```python
from build123d import *

# Parameters (mm, degrees)
F0_R     = 100
F0_R_2   = 16
F1_DEPTH = 60
F2_R     = 5
F2_R_2   = 16
F3_DEPTH = 10


with BuildPart() as f1:
    # F0 (on Right) → F1 (new body)
    with BuildSketch(Plane.YZ):
        Circle(F0_R)
        Circle(F0_R_2, mode=Mode.SUBTRACT)
    extrude(amount=F1_DEPTH)

    # F2 (on face) → F3 (join)
    with BuildSketch(Plane.YZ.offset(60)):
        with BuildLine():
            Line((-83.269003, -55.37394), (-94.310643, -89.356614))
            ThreePointArc((-94.310643, -89.356614), (-90.759655, -111.776671), (-70.53423, -122.082039))
            Line((-70.53423, -122.082039), (70.53423, -122.082039))
            ThreePointArc((70.53423, -122.082039), (90.759655, -111.776671), (94.310643, -89.356614))
            Line((94.310643, -89.356614), (83.269003, -55.37394))
            ThreePointArc((83.269003, -55.37394), (73.531721, -67.772311), (61.966923, -78.486307))
            ThreePointArc((61.966923, -78.486307), (62.5702, -79.627649), (62.778525, -80.901699))
            ThreePointArc((62.778525, -80.901699), (59.976487, -84.718097), (55.496082, -83.187649))
            ThreePointArc((55.496082, -83.187649), (0, -100), (-55.496082, -83.187649))
            ThreePointArc((-55.496082, -83.187649), (-61.129666, -84.137767), (-61.966923, -78.486307))
            ThreePointArc((-61.966923, -78.486307), (-73.531721, -67.772311), (-83.269003, -55.37394))
        make_face()
        with Locations((-70.53423, -97.082039)):
            Circle(F2_R, mode=Mode.SUBTRACT)
        with Locations((70.53423, -97.082039)):
            Circle(F2_R, mode=Mode.SUBTRACT)
        with BuildLine():
            Line((-34.818053, 93.74275), (-83.269003, -55.37394))
            ThreePointArc((-83.269003, -55.37394), (-73.531721, -67.772311), (-61.966923, -78.486307))
            ThreePointArc((-61.966923, -78.486307), (-57.504475, -77.110025), (-54.778525, -80.901699))
            ThreePointArc((-54.778525, -80.901699), (-54.962128, -82.099661), (-55.496082, -83.187649))
            ThreePointArc((-55.496082, -83.187649), (0, -100), (55.496082, -83.187649))
            ThreePointArc((55.496082, -83.187649), (56.427384, -77.665631), (61.966923, -78.486307))
            ThreePointArc((61.966923, -78.486307), (73.531721, -67.772311), (83.269003, -55.37394))
            Line((83.269003, -55.37394), (34.818053, 93.74275))
            ThreePointArc((34.818053, 93.74275), (0, 100), (-34.818053, 93.74275))
        make_face()
        Circle(F2_R_2, mode=Mode.SUBTRACT)
        with BuildLine():
            Line((-23.776413, 127.725425), (-34.818053, 93.74275))
            ThreePointArc((-34.818053, 93.74275), (0, 100), (34.818053, 93.74275))
            Line((34.818053, 93.74275), (23.776413, 127.725425))
            ThreePointArc((23.776413, 127.725425), (0, 145), (-23.776413, 127.725425))
        make_face()
        with Locations((0, 120)):
            Circle(F2_R, mode=Mode.SUBTRACT)
        Circle(F2_R_2)
    extrude(amount=F3_DEPTH)

    # F4: F1 across face


with BuildPart() as f1_1:
    add(f1.part)
    add(f1.part.mirror(Plane(origin=(0, 0, 0), x_dir=(0, 1, 0), z_dir=(-1, 0, 0))))


solid = f1_1.part
```
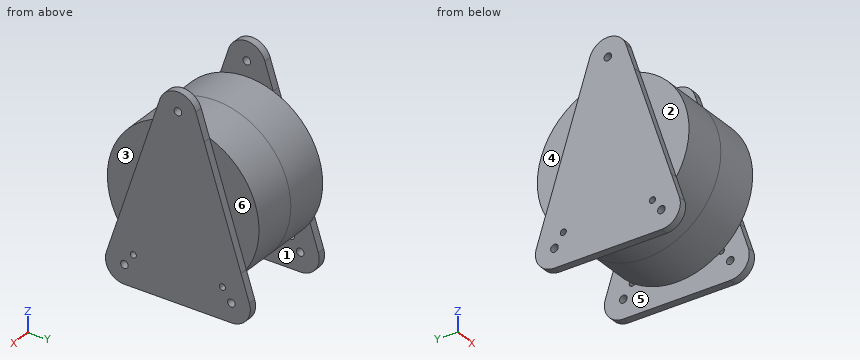
Geometry: final body of the model. Coordinates: model frame, mm. Face numbers are marked on the shaded views. A direction names the side the tool comes from. Coordinates: 2 decimals unless noted, no trailing zeros. Order: outer loops, then holes, each group sorted by start corner. A loop starts at its lowest first (then second) coordinate and runs counter-clockwise, first axis right, second up. Notation, with made-up numbers: (-30.75, 0.25) -> (3.25, 0.25) arc R21 cw to (3.25, 9.25) -> close; hole circle Ø11 at (21, 2). An arc over 180 degrees is marked (long way). Answer in a Markdown table with one row per item.
Item 1: Access query for the marked faces 1, 2 and 3. Directions: +Z, -Z, +X, -X, +Y, -Y. A direction counts if a zero-diameter tool reaches every point of the face in a straight line with its end or side. Return the directions, or none.
Return value:
| item | result |
|---|---|
| face 1 | -Z |
| face 2 | +Z, -X, -Y |
| face 3 | +Z, +X, -Y |
Item 2: Draft query along X for the marked faces 4, 5 and 6. Return one class per face: released by +X, released by -X, zero draft, split by the parting line, or undercut.
Return value:
| item | result |
|---|---|
| face 4 | released by -X |
| face 5 | undercut |
| face 6 | released by +X |
Item 3: Contact query for flat-ended pins moving along their axis: P1, Ø1.9, axis at y = -59, z = -80, coming from the -X side; P2, Ø5, axis at x = 8, z = 77, coming from the +Y side; P3, Ø5, axis at x = -2.5, y = -70, coming from the +Z side; P4, Ø9, axis at y = 0, z = 120, coming from the -X side. Output: stop coordinate, or through.
Return value:
| item | result |
|---|---|
| P1 | stops at x = -60 |
| P2 | stops at y = 66.71 |
| P3 | stops at z = 73.78 |
| P4 | passes through |
Item 4: Section C-C on x = -6. Output: boundary loops of the cut face in (y, z), plus the area to 3 significant figures.
Return value:
| item | result |
|---|---|
| outline | circle Ø200 at (0, 0); hole circle Ø32 at (0, 0) |
| area | 30,600 mm² |
Item 5: Section A-A on y = 0. Output: boundary loops of the cut face in (x, z), plus the area to 3 significant figures.
Return value:
| item | result |
|---|---|
| outline | (-70, -122.08) -> (-60, -122.08) -> (-60, -100) -> (60, -100) -> (60, -122.08) -> (70, -122.08) -> (70, 115) -> (60, 115) -> (60, 100) -> (-60, 100) -> (-60, 115) -> (-70, 115) -> close; (-70, 125) -> (-60, 125) -> (-60, 145) -> (-70, 145) -> close; (60, 125) -> (70, 125) -> (70, 145) -> (60, 145) -> close; hole (-60, -16) -> (60, -16) -> (60, 16) -> (-60, 16) -> close |
| area | 25,300 mm² |
Item 6: Section D-D on z = 0. Output: boundary loops of the cut face in (x, y).
Return value:
| item | result |
|---|---|
| outline | (-70, -65.28) -> (-60, -65.28) -> (-60, -100) -> (60, -100) -> (60, -65.28) -> (70, -65.28) -> (70, 65.28) -> (60, 65.28) -> (60, 100) -> (-60, 100) -> (-60, 65.28) -> (-70, 65.28) -> close; hole (-60, -16) -> (60, -16) -> (60, 16) -> (-60, 16) -> close |
Item 7: Ray query, L1, parallel to X at y = -85.5, z = -70.5; L2, parallel to Z at x = 19, y = 0; L3, parallel to X at y = 62, z = 11.5. Return the intervals inside material, ascending.
Return value:
| item | result |
|---|---|
| L1 | x = -70 to -60, 60 to 70 |
| L2 | z = -100 to -16, 16 to 100 |
| L3 | x = -60 to 60 |
Item 8: Section B-B on z = 120. Output: boundary loops of the cut face in (x, y).
Return value:
| item | result |
|---|---|
| outline | (-70, -26.29) -> (-60, -26.29) -> (-60, -5) -> (-70, -5) -> close; (-70, 5) -> (-60, 5) -> (-60, 26.29) -> (-70, 26.29) -> close; (60, -26.29) -> (70, -26.29) -> (70, -5) -> (60, -5) -> close; (60, 5) -> (70, 5) -> (70, 26.29) -> (60, 26.29) -> close |
